```python
from build123d import *

# Parameters (mm, degrees)
BOSS_EXTRUDE1_DEPTH                                  = 35
CUT_EXTRUDE1_DEPTH                                   = 30
SKETCH3_R                                            = 20.000000000000007
CUT_EXTRUDE2_DEPTH                                   = 52.96152422706633
M4_TAPPED_HOLE1_D                                    = 3.3
M4_TAPPED_HOLE1_DEPTH                                = 10.1
M4_TAPPED_HOLE1_TIP                                  = 0.9914200213954745
BOSS_EXTRUDE2_DEPTH                                  = 5
CBORE_FOR_M4_HEXAGON_SOCKET_HEAD_CAP_SCR_D           = 4.5
CBORE_FOR_M4_HEXAGON_SOCKET_HEAD_CAP_SCR_CBORE_D     = 8
CBORE_FOR_M4_HEXAGON_SOCKET_HEAD_CAP_SCR_CBORE_DEPTH = 1
CHAMFER1_SIZE                                        = 2
CHAMFER2_START                                       = 32.908965344
CHAMFER2_OUTLINE_W                                   = 7.000000000000002
CHAMFER2_OUTLINE_H                                   = 7.0000000000000036
CHAMFER2_DEPTH                                       = 3.091034656
MIRROR1_START                                        = 32.908965344
MIRROR1_AT_THE_SECOND_PLANE_COPY_1_SKETC_W           = 7.000000000000002
MIRROR1_AT_THE_SECOND_PLANE_COPY_1_SKETC_H           = 7.0000000000000036
MIRROR1_AT_THE_SECOND_PLANE_COPY_1_DEPTH             = 3.091034656
CHAMFER3_SIZE                                        = 1
CHAMFER4_SIZE                                        = 3


with BuildPart() as part:
    # Sketch1 → Boss-Extrude1 (new body)
    with BuildSketch(Plane.XY):
        Polygon((-29.999999999999993, 30), (30, 30), (30.000000000000014, -30), (-29.999999999999986, -30), align=None)
    extrude(amount=BOSS_EXTRUDE1_DEPTH)

    # Sketch2 → Cut-Extrude1 (cut)
    with BuildSketch(Plane.XY.offset(35)):
        with BuildLine():
            Line((0, 20.000000000000004), (30.00000000000001, 20.000000000000004))
            Line((30.00000000000001, 20.000000000000004), (30, -20.000000000000004))
            Line((30, -20.000000000000004), (0, -20.000000000000004))
            ThreePointArc((0, -20.000000000000004), (-20.000000000000004, 2.45e-15), (0, 20.000000000000004))
        make_face()
    extrude(amount=-CUT_EXTRUDE1_DEPTH, mode=Mode.SUBTRACT)

    # Sketch3 → Cut-Extrude2 (cut, through all)
    with BuildSketch(Plane.XY.offset(5.000000000000004)):
        Circle(SKETCH3_R)
    extrude(amount=-CUT_EXTRUDE2_DEPTH, mode=Mode.SUBTRACT)

    # M4 Tapped Hole1
    with Locations(Plane(origin=(0, 0, 0), x_dir=(-1, 0, 0), z_dir=(0, 0, -1))):
        with Locations((-25, 25), (25, 25), (25, -25), (-25, -25)):
            Hole(M4_TAPPED_HOLE1_D / 2, depth=M4_TAPPED_HOLE1_DEPTH)
            with Locations((0, 0, -(M4_TAPPED_HOLE1_DEPTH + M4_TAPPED_HOLE1_TIP / 2))):  # 118° drill point
                Cone(0, M4_TAPPED_HOLE1_D / 2, M4_TAPPED_HOLE1_TIP, mode=Mode.SUBTRACT)

    # Sketch7 → Boss-Extrude2 (add)
    with BuildSketch(Plane.XY.offset(35)):
        Polygon((-29.999999999999993, 30), (30, 29.999999999999993), (30, 40), (-29.999999999999993, 40), align=None)
        Polygon((30, -29.999999999999993), (30, -40), (-29.999999999999993, -40), (-29.999999999999993, -30), align=None)
    extrude(amount=-BOSS_EXTRUDE2_DEPTH)

    # CBORE for M4 Hexagon socket head cap screws1 (through all)
    with Locations(Plane(origin=(0, 0, 30.000000000000004), x_dir=(-1, 0, 0), z_dir=(0, 0, -1))):
        with Locations((-25, 35), (-25, -35), (25, -35), (25, 35)):
            CounterBoreHole(CBORE_FOR_M4_HEXAGON_SOCKET_HEAD_CAP_SCR_D / 2, CBORE_FOR_M4_HEXAGON_SOCKET_HEAD_CAP_SCR_CBORE_D / 2, CBORE_FOR_M4_HEXAGON_SOCKET_HEAD_CAP_SCR_CBORE_DEPTH)

    # Chamfer1
    chamfer1_edges = [part.edges().sort_by_distance(p)[0] for p in [
        (-29.999999999999993, 40, 32.5),
        (30, 40, 32.5),
        (30, -40, 32.5),
        (-29.999999999999993, -40, 32.5),
    ]]
    chamfer(chamfer1_edges, length=CHAMFER1_SIZE)

    # Chamfer2: read off the stored shape, not the designer's step
    # Chamfer2 outline → Chamfer2 (cut)
    with BuildSketch(Plane(origin=(0, 0, 0), x_dir=(0.8164965809277258, -0.40824829046386313, 0.40824829046386313), z_dir=(0.5773502691896258, 0.5773502691896258, -0.5773502691896258)).offset(CHAMFER2_START)):
        with Locations((11.5, -21.5)):
            Rectangle(CHAMFER2_OUTLINE_W, CHAMFER2_OUTLINE_H)
    chamfer2 = extrude(amount=CHAMFER2_DEPTH, mode=Mode.SUBTRACT)

    # Mirror1: Chamfer2 across plane
    add(chamfer2.mirror(Plane(origin=(0, 0, 0), x_dir=(0, 0, 1), z_dir=(1, 0, 0))), mode=Mode.SUBTRACT)

    # Mirror1 at the second plane: Chamfer2 across plane
    add(chamfer2.mirror(Plane.ZX), mode=Mode.SUBTRACT)

    # Mirror1 at the second plane copy 1 sketc → Mirror1 at the second plane copy 1 (cut)
    with BuildSketch(Plane(origin=(0, 0, 0), x_dir=(-0.8164965809277258, 0.40824829046386313, 0.40824829046386313), z_dir=(-0.5773502691896258, -0.5773502691896258, -0.5773502691896258)).offset(MIRROR1_START)):
        with Locations((11.5, -21.5)):
            Rectangle(MIRROR1_AT_THE_SECOND_PLANE_COPY_1_SKETC_W, MIRROR1_AT_THE_SECOND_PLANE_COPY_1_SKETC_H)
    extrude(amount=MIRROR1_AT_THE_SECOND_PLANE_COPY_1_DEPTH, mode=Mode.SUBTRACT)

    # Chamfer3
    chamfer3_edges = [part.edges().sort_by_distance(p)[0] for p in [
        (-20.000000000000007, 2.45e-15, 0),
    ]]
    chamfer(chamfer3_edges, length=CHAMFER3_SIZE)

    # Chamfer4
    # the kernel refuses this chamfer: 3 mm, written as the material it adds along each edge
    with BuildSketch(Plane(origin=(-13.115583238626146, 20.000000000000004, 5), x_dir=(0, -1, 0), z_dir=(1, 0, 0))) as chamfer4_piece_1_section:
        Polygon((CHAMFER4_SIZE, 0), (0, -CHAMFER4_SIZE), (0, 0), align=None)
    chamfer4_piece_1 = extrude(amount=43.11558323862616, mode=Mode.PRIVATE)
    chamfer4_piece_1 = chamfer4_piece_1 - Plane(origin=(0, 0, 5), x_dir=(1, 0, 0), z_dir=(0, 0, 1)) * Cylinder(20.000000000000007, 99, mode=Mode.PRIVATE)
    add(chamfer4_piece_1)
    with BuildSketch(Plane(origin=(30, -20.000000000000004, 5), x_dir=(0, 0, 1), z_dir=(-1, 0, 0))) as chamfer4_piece_2_section:
        Polygon((CHAMFER4_SIZE, 0), (0, CHAMFER4_SIZE), (0, 0), align=None)
    chamfer4_piece_2 = extrude(amount=43.11558323862615, mode=Mode.PRIVATE)
    chamfer4_piece_2 = chamfer4_piece_2 - Plane(origin=(0, 0, 5), x_dir=(1, 0, 0), z_dir=(0, 0, 1)) * Cylinder(20.000000000000007, 99, mode=Mode.PRIVATE)
    add(chamfer4_piece_2)


solid = part.part
```
Model file for the job. Use its own axes, mm. A direction names the side the tool comes from. Give positions to 0.01 mm unless a question says otherwise; leave off trailing zeros. Loops run counter-clockwise (first coordinate to the right, second up) from the corner with the lowest first, then second, coordinate; pieces in that order, holes last. Notation, with made-up numbers: (-34, 56.5) -> (10, 56.5) arc R16 ccw to (10, 73.5) -> close; hole circle Ø4 at (52, -22). An arc over 180 degrees is marked (long way). Use CSV: the item, a comma, the result in double quotes. Start each with the question number.
1) Flat gauge pins, fed straight in: pin 1 Ø2 at (x, z) = (21.5, 25.5) entering from -Y; pin 2 Ø6 at (x, y) = (16.5, 5) entering from +Z; pin 3 Ø2.5 at (x, y) = (-23.5, 37) entering from -Z. Where does each tip first touch, or does it go through?
2) Mould opens along Y. For faces 6 (the flat face through (-27, -37, 31)), 7 (the flat face through (7, 20, 0)), 8 (the flat face through (0, 30, 15)) say: released by +Y, released by -Y, zero draft, split by the parting line, or undercut.
3) Wall check: line 1 (X direction, y = 25, z = 5.75); line 2 (Y direction, x = -25, z = 31.9). Give the ranges that are in metal, low to high.
4) Slice it at A-A on y = 35. Give the cut face in (x, z).
5) Slice it at B-B on z = 29. Give the cut face in (x, y).
6) Slice it at C-C on z = 4. Give the cut face in (x, y), plus the area to 3 significant figures.
7) Tool access for faces 1 (the flat face through (19, -19, 7)), 2 (the cylindrical face through (26.21, -33.103, 33.028)), 3 (the flat face through (0, 35, 30)), 4 (the cylindrical face through (25.521, 38.966, 30.493)), 5 (the flat face through (-29, -29, 1)): list every direction of +Z, -Z, +X, -X, +Y, -Y with a clear straight run to the whole face (end or side of a thin tool).
Computed values:
1,pin 1,"stops at y = -30"
1,pin 2,"stops at z = 5"
1,pin 3,"stops at z = 31"
2,face 6,"undercut"
2,face 7,"zero draft"
2,face 8,"released by +Y"
3,line 1,"x = -30 to -26.65, -23.35 to 23.35, 26.65 to 30"
3,line 2,"y = -40 to -37.25, -32.75 to 32.75, 37.25 to 40"
4,outline,"(-30, 30) -> (-29, 30) -> (-29, 31) -> (-27.25, 31) -> (-27.25, 35) -> (-30, 35) -> close; (-22.75, 31) -> (-21, 31) -> (-21, 30) -> (21, 30) -> (21, 31) -> (22.75, 31) -> (22.75, 35) -> (-22.75, 35) -> close; (27.25, 31) -> (29, 31) -> (29, 30) -> (30, 30) -> (30, 35) -> (27.25, 35) -> close"
5,outline,"(-30, -30) -> (30, -30) -> (30, -20) -> (0, -20) arc R20 cw to (0, 20) -> (30, 20) -> (30, 30) -> (-30, 30) -> close"
6,outline,"(-30, -30) -> (30, -30) -> (30, 30) -> (-30, 30) -> close; hole circle Ø3.3 at (-25, -25); hole circle Ø3.3 at (-25, 25); hole circle Ø40 at (0, 0); hole circle Ø3.3 at (25, -25); hole circle Ø3.3 at (25, 25)"
6,area,"2,310 mm^2"
7,face 1,"+Z, +X"
7,face 2,"+Z, -Z"
7,face 3,"-Z, +X, -X, +Y"
7,face 4,"-Z"
7,face 5,"-Z, -X, -Y"
